```python
from build123d import *

# Parameters (mm, degrees)
SKETCH_1_R          = 2.6
EXTRUDE_1_DEPTH     = 3
CUT_EXTRUDE_START   = -3
CUT_EXTRUDE_1_DEPTH = 3
SKETCH_3_R          = 1.6
CUT_EXTRUDE_2_DEPTH = 3
FILLET_1_R          = 1
SKETCH_4_R          = 1.75
CUT_EXTRUDE_3_DEPTH = 10
SKETCH_5_W          = 40
SKETCH_5_H          = 5.4
EXTRUDE_2_DEPTH     = 3
SKETCH_6_R          = 1.25
CUT_EXTRUDE_4_DEPTH = 4
FILLET_2_R          = 2


with BuildPart() as part:
    # 草图1 → 凸台-拉伸1 (new body)
    with BuildSketch(Plane.XY):
        with BuildLine():
            Line((-35, -27.5), (27.5, -27.5))
            ThreePointArc((27.5, -27.5), (32.803300859, -25.303300859), (35, -20))
            Line((35, -20), (35, 20))
            ThreePointArc((35, 20), (32.803300859, 25.303300859), (27.5, 27.5))
            Line((27.5, 27.5), (-35, 27.5))
            Line((-35, 27.5), (-35, -27.5))
        make_face()
        with Locations((27.5, 20)):
            Circle(SKETCH_1_R, mode=Mode.SUBTRACT)
        with Locations(Location((27.5, -20, 0), (0, 0, 180))):
            Circle(SKETCH_1_R, mode=Mode.SUBTRACT)
    extrude(amount=EXTRUDE_1_DEPTH)

    # 草图2 → 切除-拉伸1 (cut)
    with BuildSketch(Plane.XY.offset(3).offset(CUT_EXTRUDE_START)):
        with BuildLine():
            Line((-35, 12.5), (-5, 12.5))
            Line((-5, 12.5), (24.213483146, 26.741573034))
            ThreePointArc((24.213483146, 26.741573034), (25.8135537, 27.307933968), (27.5, 27.5))
            Line((27.5, 27.5), (27.5, 37.5))
            Line((27.5, 37.5), (-35, 37.5))
            Line((-35, 37.5), (-35, 12.5))
        make_face()
    extrude(amount=CUT_EXTRUDE_1_DEPTH, mode=Mode.SUBTRACT)

    # 草图3 → 切除-拉伸2 (cut)
    with BuildSketch(Plane.XY.offset(3)):
        with Locations((-20, 2.5)):
            Circle(SKETCH_3_R)
        with Locations(Location((5, 2.5, 0), (0, 0, 180))):
            Circle(SKETCH_3_R)
        with Locations((5, -17.5)):
            Circle(SKETCH_3_R)
        with Locations(Location((-20, -17.5, 0), (0, 0, 180))):
            Circle(SKETCH_3_R)
    extrude(amount=-CUT_EXTRUDE_2_DEPTH, mode=Mode.SUBTRACT)

    # 圆角1
    fillet_1_edges = [part.edges().sort_by_distance(p)[0] for p in [
        (-35, -27.5, 1.5),
        (-35, 12.5, 1.5),
    ]]
    fillet(fillet_1_edges, radius=FILLET_1_R)

    # 草图4 → 切除-拉伸3 (cut)
    with BuildSketch(Plane.XY.offset(3)):
        with Locations((-2.5, 0)):
            Circle(SKETCH_4_R)
        with Locations((-12.5, 0)):
            Circle(SKETCH_4_R)
        with Locations((-12.5, -15)):
            Circle(SKETCH_4_R)
        with Locations((-2.5, -15)):
            Circle(SKETCH_4_R)
    extrude(amount=-CUT_EXTRUDE_3_DEPTH, mode=Mode.SUBTRACT)

    # 草图5 → 凸台-拉伸2 (add)
    with BuildSketch(Plane(origin=(0, 0, 0), x_dir=(-1, 0, 0), z_dir=(0, 0, -1))):
        with Locations((15, -29.2)):
            Rectangle(SKETCH_5_W, SKETCH_5_H)
    extrude(amount=-EXTRUDE_2_DEPTH)

    # 草图6 → 切除-拉伸4 (cut)
    with BuildSketch(Plane(origin=(0, 0, 0), x_dir=(-1, 0, 0), z_dir=(0, 0, -1))):
        with Locations((30, -28.95)):
            Circle(SKETCH_6_R)
        with Locations((10, -28.95)):
            Circle(SKETCH_6_R)
    extrude(amount=-CUT_EXTRUDE_4_DEPTH, mode=Mode.SUBTRACT)

    # 圆角2
    fillet_2_edges = [part.edges().sort_by_distance(p)[0] for p in [
        (5, -27.5, 1.5),
        (5, -31.9, 1.5),
        (-35, -31.9, 1.5),
        (-5, 12.5, 1.5),
    ]]
    fillet(fillet_2_edges, radius=FILLET_2_R)


solid = part.part
```
CAD build for the part. Positions are in the model's coordinates, mm. A direction names the side the tool comes from. Round coordinates to 2 decimals unless told otherwise and drop trailing zeros. Loops run counter-clockwise (first coordinate to the right, second up) from the corner with the lowest first, then second, coordinate; pieces in that order, holes last. Notation, with made-up numbers: M -39,-20.75 L -4,-20.75 A34 ccw -4,17.25 Z; hole C 23.25,60 d9. An arc over 180 degrees is marked long. Return JSON: item names as keys, results as strings. Group by question number.
(1) Saw through at B-B, the plane z = 0.8. Give the number of separate pieces and of enclosed holes in the cut face, and give its area (3 significant figures).
(2) Mould opens along Y. For faces 3 (the cylindrical face through (27.838, -22.578, 1.479)), 4 (the flat face through (9.613, 19.624, 1.479)), 5 (the cylindrical face through (-34.4, -31.33, 1.52)) say: +Y half, -Y half, draft (parallel to the pull), parting line (faces both ways), or undercut.
(3) Wall check: probe 1 along Y at (x, z) = (-12.5, 0.7); probe 2 along Y at (x, z) = (27.5, 1.1); probe 3 along X at (y, z) = (-20, 1.6). Give the ranges that are in metal, low to high. Write a range as [from, to].
(4) Saw through at C-C, the plane x = -12.5. List the corners of the cut face in (y, z).
(5) Tool access for faces 1 (the flat face through (-20, 12.5, 1)), 2 (the cylindrical face through (5.57, -28.1, 1.52)): list every direction of +Z, -Z, +X, -X, +Y, -Y with a clear straight run to the whole face (end or side of a thin tool).
(6) Saw through at D-D, the plane x = -3. List the corners of the cut face in (y, z) (3 decimals), and give its area (3 significant figures).
(7) Saw through at A-A, the plane x = -30. List the corners of the cut face in (y, z), and give its area (3 significant figures).
Answer list:
{
 "1": {"separate pieces": "1", "enclosed holes": "12", "area": "3,200 mm2"},
 "2": {"face 3": "undercut", "face 4": "+Y half", "face 5": "-Y half"},
 "3": {"probe 1": "[-31.9, -16.75], [-13.25, -1.75], [1.75, 12.5]", "probe 2": "[-27.5, -22.6], [-17.4, 17.4], [22.6, 27.5]", "probe 3": "[-35, 24.9], [30.1, 35]"},
 "4": {"outline": "M -31.9,0 L -16.75,0 L -16.75,3 L -31.9,3 Z; M -13.25,0 L -1.75,0 L -1.75,3 L -13.25,3 Z; M 1.75,0 L 12.5,0 L 12.5,3 L 1.75,3 Z"},
 "5": {"face 1": "+Z, -Z, -X, +Y", "face 2": "+Z, -Z, +X, -Y"},
 "6": {"outline": "M -31.9,0 L -16.677,0 L -16.677,3 L -31.9,3 Z; M -13.323,0 L -1.677,0 L -1.677,3 L -13.323,3 Z; M 1.677,0 L 13.475,0 L 13.475,3 L 1.677,3 Z", "area": "116 mm2"},
 "7": {"outline": "M -31.9,0 L -30.2,0 L -30.2,3 L -31.9,3 Z; M -27.7,0 L 12.5,0 L 12.5,3 L -27.7,3 Z", "area": "126 mm2"}
}
